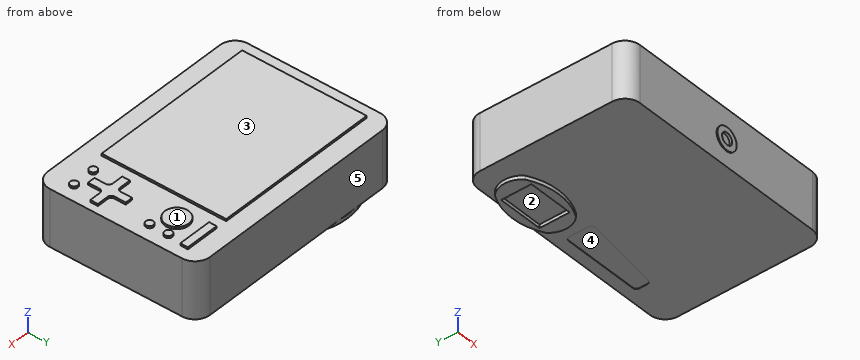
```python
from build123d import *

# Parameters (mm, degrees)
EXTRUDE1_DEPTH     = 1
EXTRUDE9_DEPTH     = 21.8125
EXTRUDE10_DEPTH    = 1
SKETCH14_R         = 1.5875
SKETCH14_R_2       = 5.020115786
SKETCH14_W         = 69.85
SKETCH14_H         = 52.3875
SKETCH14_W_2       = 14.2875
SKETCH14_H_2       = 3.175
EXTRUDE12_DEPTH    = 0.9
CUT_EXTRUDE5_DEPTH = 0.2
EXTRUDE13_DEPTH    = 1.5875
SKETCH17_W         = 19.05
SKETCH17_H         = 12.7
CUT_EXTRUDE6_DEPTH = 1.5
SKETCH18_R         = 4.7625
EXTRUDE14_DEPTH    = 0.4
SKETCH19_R         = 2.5
CUT_EXTRUDE7_DEPTH = 1


with BuildPart() as part:
    # Sketch1 → Extrude1 (new body)
    with BuildSketch(Plane.XY):
        with BuildLine():
            Line((-42.8625, 34.925), (42.8625, 34.925))
            ThreePointArc((42.8625, 34.925), (47.352628061, 33.065128061), (49.2125, 28.575))
            Line((49.2125, 28.575), (49.2125, -26.9875))
            ThreePointArc((49.2125, -26.9875), (47.352628061, -31.477628061), (42.8625, -33.3375))
            Line((42.8625, -33.3375), (-42.8625, -33.3375))
            ThreePointArc((-42.8625, -33.3375), (-47.352628061, -31.477628061), (-49.2125, -26.9875))
            Line((-49.2125, -26.9875), (-49.2125, 28.575))
            ThreePointArc((-49.2125, 28.575), (-47.352628061, 33.065128061), (-42.8625, 34.925))
        make_face()
    extrude(amount=EXTRUDE1_DEPTH)

    # Sketch11 → Extrude9 (add)
    with BuildSketch(Plane.XY.offset(1)):
        with BuildLine():
            Line((-42.8625, 34.925), (42.8625, 34.925))
            ThreePointArc((42.8625, 34.925), (47.352628061, 33.065128061), (49.2125, 28.575))
            Line((49.2125, 28.575), (49.2125, -26.9875))
            ThreePointArc((49.2125, -26.9875), (47.352628061, -31.477628061), (42.8625, -33.3375))
            Line((42.8625, -33.3375), (-42.8625, -33.3375))
            ThreePointArc((-42.8625, -33.3375), (-47.352628061, -31.477628061), (-49.2125, -26.9875))
            Line((-49.2125, -26.9875), (-49.2125, 28.575))
            ThreePointArc((-49.2125, 28.575), (-47.352628061, 33.065128061), (-42.8625, 34.925))
        make_face()
        with BuildLine():
            Line((-42.8625, 33.3375), (42.8625, 33.3375))
            ThreePointArc((42.8625, 33.3375), (46.230096045, 31.942596045), (47.625, 28.575))
            Line((47.625, 28.575), (47.625, -26.9875))
            ThreePointArc((47.625, -26.9875), (46.230096045, -30.355096045), (42.8625, -31.75))
            Line((42.8625, -31.75), (-42.8625, -31.75))
            ThreePointArc((-42.8625, -31.75), (-46.230096045, -30.355096045), (-47.625, -26.9875))
            Line((-47.625, -26.9875), (-47.625, 28.575))
            ThreePointArc((-47.625, 28.575), (-46.230096045, 31.942596045), (-42.8625, 33.3375))
        make_face(mode=Mode.SUBTRACT)
    extrude(amount=EXTRUDE9_DEPTH)

    # Sketch13 → Extrude10 (add)
    with BuildSketch(Plane.XY.offset(22.8125)):
        with BuildLine():
            Line((-42.8625, 34.925), (42.8625, 34.925))
            ThreePointArc((42.8625, 34.925), (47.352628061, 33.065128061), (49.2125, 28.575))
            Line((49.2125, 28.575), (49.2125, -26.9875))
            ThreePointArc((49.2125, -26.9875), (47.352628061, -31.477628061), (42.8625, -33.3375))
            Line((42.8625, -33.3375), (-42.8625, -33.3375))
            ThreePointArc((-42.8625, -33.3375), (-47.352628061, -31.477628061), (-49.2125, -26.9875))
            Line((-49.2125, -26.9875), (-49.2125, 28.575))
            ThreePointArc((-49.2125, 28.575), (-47.352628061, 33.065128061), (-42.8625, 34.925))
        make_face()
    extrude(amount=EXTRUDE10_DEPTH)

    # Sketch14 → Extrude12 (add)
    with BuildSketch(Plane.XY.offset(23.8125)):
        with Locations(Location((42.8625, 17.4625, 0), (0, 0, 180))):
            Circle(SKETCH14_R)
        with Locations(Location((42.8625, 9.525, 0), (0, 0, 180))):
            Circle(SKETCH14_R)
        with Locations(Location((34.925, 14.2875, 0), (0, 0, 180))):
            Circle(SKETCH14_R_2)
        with Locations(Location((33.3375, -22.225, 0), (0, 0, 180))):
            Circle(SKETCH14_R)
        with Locations(Location((42.8625, -22.225, 0), (0, 0, 180))):
            Circle(SKETCH14_R)
        with BuildLine():
            Line((36.5125, -7.9375), (36.5125, -3.175))
            Line((36.5125, -3.175), (39.6875, -3.175))
            Line((39.6875, -3.175), (39.6875, -7.9375))
            ThreePointArc((39.6875, -7.9375), (40.152467985, -9.060032015), (41.275, -9.525))
            Line((41.275, -9.525), (46.0375, -9.525))
            Line((46.0375, -9.525), (46.0375, -12.7))
            Line((46.0375, -12.7), (41.275, -12.7))
            ThreePointArc((41.275, -12.7), (40.152467985, -13.164967985), (39.6875, -14.2875))
            Line((39.6875, -14.2875), (39.6875, -19.05))
            Line((39.6875, -19.05), (36.5125, -19.05))
            Line((36.5125, -19.05), (36.5125, -14.2875))
            ThreePointArc((36.5125, -14.2875), (36.047532015, -13.164967985), (34.925, -12.7))
            Line((34.925, -12.7), (30.1625, -12.7))
            Line((30.1625, -12.7), (30.1625, -9.525))
            Line((30.1625, -9.525), (34.925, -9.525))
            ThreePointArc((34.925, -9.525), (36.047532015, -9.060032015), (36.5125, -7.9375))
        make_face()
        with Locations((-9.525, 0.79375)):
            Rectangle(SKETCH14_W, SKETCH14_H)
        with Locations((37.30625, 25.4)):
            Rectangle(SKETCH14_W_2, SKETCH14_H_2)
    extrude(amount=EXTRUDE12_DEPTH)

    # Sketch15 → Cut-Extrude5 (cut)
    with BuildSketch(Plane(origin=(0, 0, 0), x_dir=(-1, 0, 0), z_dir=(0, 0, -1))):
        with BuildLine():
            Line((3.175, 30.1625), (-28.575, 30.1625))
            ThreePointArc((-28.575, 30.1625), (-29.697532015, 29.697532015), (-30.1625, 28.575))
            Line((-30.1625, 28.575), (-30.1625, 25.4))
            ThreePointArc((-30.1625, 25.4), (-29.697532015, 24.277467985), (-28.575, 23.8125))
            Line((-28.575, 23.8125), (3.175, 19.05))
            ThreePointArc((3.175, 19.05), (4.297532015, 19.514967985), (4.7625, 20.6375))
            Line((4.7625, 20.6375), (4.7625, 28.575))
            ThreePointArc((4.7625, 28.575), (4.297532015, 29.697532015), (3.175, 30.1625))
        make_face()
    extrude(amount=-CUT_EXTRUDE5_DEPTH, mode=Mode.SUBTRACT)

    # Sketch16 → Extrude13 (add)
    with BuildSketch(Plane(origin=(0, 0, 0), x_dir=(-1, 0, 0), z_dir=(0, 0, -1))):
        with BuildLine():
            ThreePointArc((12.7, 31.75), (25.4, 35.122668351), (38.1, 31.75))
            ThreePointArc((38.1, 31.75), (40.730256121, 25.4), (38.1, 19.05))
            ThreePointArc((38.1, 19.05), (25.4, 15.677331649), (12.7, 19.05))
            ThreePointArc((12.7, 19.05), (10.069743879, 25.4), (12.7, 31.75))
        make_face()
    extrude(amount=EXTRUDE13_DEPTH)

    # Sketch17 → Cut-Extrude6 (cut)
    with BuildSketch(Plane(origin=(0, 0, -1.5875), x_dir=(-1, 0, 0), z_dir=(0, 0, -1))):
        with Locations((25.4, 25.4)):
            Rectangle(SKETCH17_W, SKETCH17_H)
    extrude(amount=-CUT_EXTRUDE6_DEPTH, mode=Mode.SUBTRACT)

    # Sketch18 → Extrude14 (add)
    with BuildSketch(Plane.XZ.offset(33.3375)):
        with Locations(Location((0, 11.1125, 0), (0, 0, 180))):
            Circle(SKETCH18_R)
    extrude(amount=EXTRUDE14_DEPTH)

    # Sketch19 → Cut-Extrude7 (cut)
    with BuildSketch(Plane.XZ.offset(33.7375)):
        with Locations((0, 11.1125)):
            Circle(SKETCH19_R)
    extrude(amount=-CUT_EXTRUDE7_DEPTH, mode=Mode.SUBTRACT)


solid = part.part
```
Part model, mm, in its own coordinate system. Face numbers are marked on the shaded views. A direction names the side the tool comes from. Coordinates: 2 decimals unless noted, no trailing zeros. Return JSON: item names as keys, results as strings. Group by question number.
Item 1: Which spindle directions (+Z, -Z, +X, -X, +Y, -Y) get a long thin tool onto all of the face, cutting with end or side? Do the marked faces 1 and 2. Say none if no direction does.
Item 2: Pin check, flat tips, straight feed: pin 1 (4 mm diameter, centred on x = 24.5, y = 24.5, fed in from -Z); pin 2 (1 mm diameter, centred on x = -2, z = 5, fed in from -Y); pin 3 (1 mm diameter, centred on x = 39, z = 24.5, fed in from -Y). Stop position of each tip, or through.
Item 3: Pull direction Y, two halves, no side cores. Call the marked faces 3, 4 and 5: pulls with the +Y half, pulls with the -Y half, needs draft (parallel to the pull), parting line crosses it, or undercut.
Item 4: Drill centre lines: probe 1 along Z at (x, y) = (-7, 26); probe 2 along Z at (x, y) = (28, 13); probe 3 along X at (y, z) = (-15, 9.75) (1 decimal). Where is each one in solid material? Low to high. Write a range as from..to.
Check values:
{
 "1": {"face 1": "+Z, +X, -X, +Y, -Y", "face 2": "-Z"},
 "2": {"pin 1": "stops at z = 0", "pin 2": "stops at y = -33.34", "pin 3": "stops at y = -19.05"},
 "3": {"face 3": "needs draft", "face 4": "undercut", "face 5": "pulls with the +Y half"},
 "4": {"probe 1": "z = 0..1, 22.81..24.71", "probe 2": "z = 0..1, 22.81..23.81", "probe 3": "x = -49.2..-47.6, 47.6..49.2"}
}
